from build123d import *

# Parameters (mm, degrees)
SKETCH_1_R                   = 50
EXTRUDE_1_DEPTH              = 5
SKETCH_8_W                   = 26
SKETCH_8_H                   = 32.5
EXTRUDE_3_DEPTH              = 10
SKETCH_6_R                   = 6.5
CUT_EXTRUDE_1_DEPTH          = 73.284161474
HOLE_WIZARD_M2_1_D           = 2.4
HOLE_WIZARD_M2_1_CBORE_D     = 3.85
HOLE_WIZARD_M2_1_CBORE_DEPTH = 1.45
HOLE_WIZARD_M3_2_D           = 3.4
HOLE_WIZARD_M3_2_CBORE_D     = 6.05
HOLE_WIZARD_M3_2_CBORE_DEPTH = 2.2
PATTERN_CIRCULAR_1_COUNT     = 8
SKETCH_7_W                   = 3
SKETCH_7_H                   = 15
EXTRUDE_2_DEPTH              = 3
FILLET_1_R                   = 1
FILLET_1_OF_MIRROR_2_R       = 1
FILLET_2_R                   = 2.5
SKETCH_9_W                   = 5
SKETCH_9_H                   = 2
CUT_EXTRUDE_2_DEPTH          = 72.414284285


with BuildPart() as part:
    # ｽｹｯﾁ1 → ﾎﾞｽ - 押し出し1 (new body)
    with BuildSketch(Plane.XY):
        Circle(SKETCH_1_R)
    extrude(amount=EXTRUDE_1_DEPTH)

    # ｽｹｯﾁ8 → ﾎﾞｽ - 押し出し3 (add)
    with BuildSketch(Plane(origin=(0, 0, 0), x_dir=(-1, 0, 0), z_dir=(0, 0, -1))):
        with Locations((0, -7.37)):
            Rectangle(SKETCH_8_W, SKETCH_8_H)
    extrude(amount=EXTRUDE_3_DEPTH)

    # ｽｹｯﾁ6 → ｶｯﾄ - 押し出し1 (cut, through all)
    with BuildSketch(Plane.XY.offset(5)):
        Circle(SKETCH_6_R)
    extrude(amount=-CUT_EXTRUDE_1_DEPTH, mode=Mode.SUBTRACT)

    # M2 丸平ねじ用座ぐり穴1 (through all)
    with Locations(Plane.XY.offset(5)):
        with Locations((-10.5, 0), (-10.5, -21)):
            hole_wizard_m2_1 = CounterBoreHole(HOLE_WIZARD_M2_1_D / 2, HOLE_WIZARD_M2_1_CBORE_D / 2, HOLE_WIZARD_M2_1_CBORE_DEPTH)

    # ﾐﾗｰ1: M2 丸平ねじ用座ぐり穴1 across plane
    add(hole_wizard_m2_1.mirror(Plane(origin=(0, 0, 0), x_dir=(0, 0, 1), z_dir=(1, 0, 0))), mode=Mode.SUBTRACT)

    # M3 丸平ねじ用座ぐり穴2 (through all)
    with Locations(Plane.XY.offset(5)):
        with Locations((45, 0)):
            hole_wizard_m3_2 = CounterBoreHole(HOLE_WIZARD_M3_2_D / 2, HOLE_WIZARD_M3_2_CBORE_D / 2, HOLE_WIZARD_M3_2_CBORE_DEPTH)

    # 円形ﾊﾟﾀｰﾝ1: M3 丸平ねじ用座ぐり穴2 ×8 about axis
    pattern_circular_1_axis = Axis((0, 0, 0), (0, 0, 1))
    for i in range(1, PATTERN_CIRCULAR_1_COUNT):
        add(hole_wizard_m3_2.rotate(pattern_circular_1_axis, i * 360 / PATTERN_CIRCULAR_1_COUNT), mode=Mode.SUBTRACT)

    # ｽｹｯﾁ7 → ﾎﾞｽ - 押し出し2 (add)
    with BuildSketch(Plane(origin=(0, 0, 0), x_dir=(-1, 0, 0), z_dir=(0, 0, -1))):
        with Locations((26.5, 17.5)):
            Rectangle(SKETCH_7_W, SKETCH_7_H)
    extrude_2 = extrude(amount=EXTRUDE_2_DEPTH)

    # ﾌｨﾚｯﾄ1
    fillet_1_edges = [part.edges().sort_by_distance(p)[0] for p in [
        (-28, 17.5, 0),
    ]]
    fillet(fillet_1_edges, radius=FILLET_1_R)

    # ﾐﾗｰ2: ﾎﾞｽ - 押し出し2 across plane
    add(extrude_2.mirror(Plane(origin=(0, 0, 0), x_dir=(0, 0, 1), z_dir=(1, 0, 0))))

    # ﾌｨﾚｯﾄ1 of ﾐﾗｰ2
    fillet_1_of_mirror_2_edges = [part.edges().sort_by_distance(p)[0] for p in [
        (28, 17.5, 0),
    ]]
    fillet(fillet_1_of_mirror_2_edges, radius=FILLET_1_OF_MIRROR_2_R)

    # ﾌｨﾚｯﾄ2
    fillet_2_edges = [part.edges().sort_by_distance(p)[0] for p in [
        (-13, -23.62, -5),
        (-13, 8.88, -5),
        (13, 8.88, -5),
        (13, -23.62, -5),
    ]]
    fillet(fillet_2_edges, radius=FILLET_2_R)

    # ｽｹｯﾁ9 → ｶｯﾄ - 押し出し2 (cut, through all)
    with BuildSketch(Plane(origin=(0, 0, 0), x_dir=(-1, 0, 0), z_dir=(0, 0, -1))):
        with Locations((17.5, 35)):
            Rectangle(SKETCH_9_W, SKETCH_9_H)
        with Locations((17.5, 8)):
            Rectangle(SKETCH_9_W, SKETCH_9_H)
    cut_extrude_2 = extrude(amount=-CUT_EXTRUDE_2_DEPTH, mode=Mode.SUBTRACT)

    # ﾐﾗｰ3: ｶｯﾄ - 押し出し2 across plane
    add(cut_extrude_2.mirror(Plane(origin=(0, 0, 0), x_dir=(0, 0, 1), z_dir=(1, 0, 0))), mode=Mode.SUBTRACT)


solid = part.part
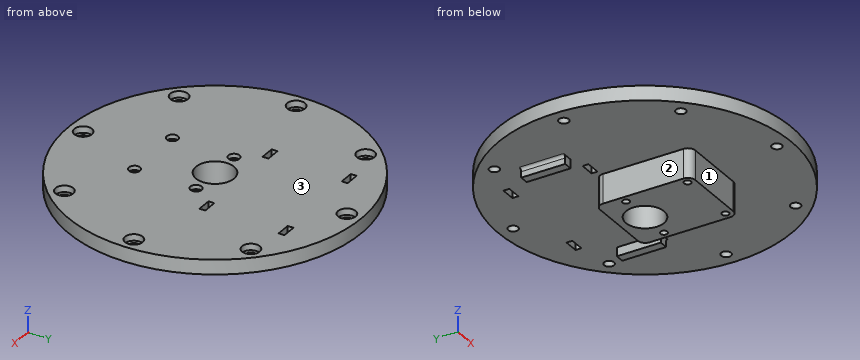
Input: part model. Units: mm. Frame: model coordinates. Face numbers are marked on the shaded views. A direction names the side the tool comes from. Give positions to 0.01 mm unless a question says otherwise; leave off trailing zeros. Write each loop counter-clockwise with the first axis right and the second up, starting at its lowest first coordinate (ties: lowest second). Pieces come first, ordered by that corner, then holes. Notation, with made-up numbers: M -28.75,4.5 L 23.25,4.5 A17 ccw 23.25,30.5 Z; hole C 72.25,-33 d10. An arc over 180 degrees is marked long. Write item = value, one per line. Start each with the question number.
1) Material intervals for line 1 along Y through (x, z) = (10.5, -0.75); line 2 along Y through (x, z) = (0.5, -2.25); line 3 along X through (y, z) = (-45, 3.8) (1 decimal), sorted ascending. Write a range as [from, to].
2) Cut plane D-D on y = 13. Return the cut outline in (x, z).
3) First-contact query: pin 1 Ø0.9 at (x, z) = (-26.5, -2) entering from +Y; pin 2 Ø5 at (x, z) = (1, -3) entering from -Y; pin 3 Ø4 at (x, y) = (19, 7) entering from -Z. Flat tips, straight axial feed; report the tip coordinate or a pass-through.
4) Reachability of the marked faces 1, 2 and 3 from +Z, -Z, +X, -X, +Y, -Y: full face, straight path, thin tool, end or side. Return the list, or none.
5) Cut plane A-A on z = -8. Return the cut outline in (x, y).
6) Cut plane B-B on y = 45. Return the cut outline in (x, z) (1 decimal).
7) Cut plane C-C on y = 0. Count the separate pieces of the cut face and the enclosed holes in it, then the cut area to 3 significant figures.
Solved:
q1.line_1 = [-23.62, -22.2], [-19.8, -1.2], [1.2, 8.88]
q1.line_2 = [-23.62, -6.48], [6.48, 8.88]
q1.line_3 = [-21.8, -3], [3, 21.8]
q2.outline = M -48.28,0 L -29,0 A1 cw -28,-1 L -28,-3 L -25,-3 L -25,0 L 25,0 L 25,-3 L 28,-3 L 28,-1 A1 cw 29,0 L 48.28,0 L 48.28,5 L -48.28,5 Z
q3.pin_1 = 25
q3.pin_2 = -23.62
q3.pin_3 = 0
q4.face_1 = -Z, +X, -X, -Y
q4.face_2 = -Z, -X, +Y, -Y
q4.face_3 = +Z, +X, -X, +Y, -Y
q5.outline = M -13,-21.12 A2.5 ccw -10.5,-23.62 L 10.5,-23.62 A2.5 ccw 13,-21.12 L 13,6.38 A2.5 ccw 10.5,8.88 L -10.5,8.88 A2.5 ccw -13,6.38 Z; hole C -10.5,-21 d2.4; hole C -10.5,0 d2.4; hole C 0,0 d13; hole C 10.5,-21 d2.4; hole C 10.5,0 d2.4
q6.outline = M -21.8,0 L -1.7,0 L -1.7,2.8 L -3,2.8 L -3,5 L -21.8,5 Z; M 1.7,0 L 21.8,0 L 21.8,5 L 3,5 L 3,2.8 L 1.7,2.8 Z
q7.separate_pieces = 6
q7.enclosed_holes = 0
q7.area = 443 mm2
